Check sheet for the modelled part. Datum: model origin and axes. Units: mm. Round coordinates to 2 decimals unless told otherwise and drop trailing zeros.
Q1. Cross-section at A-A on y = 0.9. Give the number of separate pieces and of enclosed holes in the cut face, then the cut area to 3 significant figures.
Q2. Depth check by flat-ended pin: P1, Ø3.5, axis at x = -7.07, z = 7.07, coming from the +Y side; P2, Ø5.5, axis at x = -135, z = 0, coming from the -Y side. Enter the tip coordinate at first touch or a pass-through.
Q3. Scan lines: probe 1 along X at (y, z) = (0.4, -7.5); probe 2 along X at (y, z) = (0.35, 10); probe 3 along X at (y, z) = (1.3, -9). Record each from-to range of solid material in increasing order.
from build123d import *

# Parameters (mm, degrees)
SKETCH2_R           = 1.09
SKETCH2_R_2         = 3
SKETCH2_R_3         = 6.25
BOSS_EXTRUDE1_DEPTH = 1.5
FILLET1_R           = 10
SKETCH3_R           = 1.09
CUT_EXTRUDE1_DEPTH  = 10


with BuildPart() as part:
    # Sketch2 → Boss-Extrude1 (new body)
    with BuildSketch(Plane(origin=(0, 0, 0), x_dir=(1, 0, 0), z_dir=(0, 1, 0))):
        with BuildLine():
            add(Edge.make_bspline(
                [(15.330967743, -8.438686395), (-4.328656702, -48.917065398), (-54.77019988, -54.651995587)],
                knots=[0, 0, 0, 1, 1, 1], degree=2))
            ThreePointArc((15.330967743, -8.438686395), (3.221708095, 17.200889423), (-17.345753159, -2.318371704))
            add(Edge.make_bspline(
                [(-17.345753159, -2.318371704), (-24.57230847, -34.004755189), (-64.372079348, -27.287713928)],
                knots=[0, 0, 0, 1, 1, 1], degree=2))
            add(Edge.make_bspline(
                [(-118.261066558, 5.104714216), (-107.65521746, -9.024230402), (-84.042514499, -23.671917894), (-64.372079348, -27.287713928)],
                knots=[0, 0, 0, 0, 1, 1, 1, 1], degree=3))
            ThreePointArc((-118.261066558, 5.104714216), (-148.55197352, 11.072218102), (-136.664707239, -17.420641487))
            add(Edge.make_bspline(
                [(-136.664707239, -17.420641487), (-99.493020923, -49.665084924), (-54.77019988, -54.651995587)],
                knots=[0, 0, 0, 1, 1, 1], degree=2))
        make_face()
        with Locations(Location((-141.01040764, -6.01040764, 0), (0, 0, 270))):
            Circle(SKETCH2_R, mode=Mode.SUBTRACT)
        with Locations(Location((-128.98959236, -6.01040764, 0), (0, 0, 270))):
            Circle(SKETCH2_R, mode=Mode.SUBTRACT)
        with Locations(Location((-135, 0, 0), (0, 0, 270))):
            Circle(SKETCH2_R_2, mode=Mode.SUBTRACT)
        with Locations(Location((-141.01040764, 6.01040764, 0), (0, 0, 270))):
            Circle(SKETCH2_R, mode=Mode.SUBTRACT)
        with Locations(Location((-128.98959236, 6.01040764, 0), (0, 0, 270))):
            Circle(SKETCH2_R, mode=Mode.SUBTRACT)
        with Locations(Location((-7.071067812, -7.071067812, 0), (0, 0, 270))):
            Circle(SKETCH2_R, mode=Mode.SUBTRACT)
        with Locations(Location((7.071067812, -7.071067812, 0), (0, 0, 270))):
            Circle(SKETCH2_R, mode=Mode.SUBTRACT)
        with Locations(Location((-7.071067812, 7.071067812, 0), (0, 0, 270))):
            Circle(SKETCH2_R, mode=Mode.SUBTRACT)
        with Locations(Location((0, 0, 0), (0, 0, 270))):
            Circle(SKETCH2_R_3, mode=Mode.SUBTRACT)
        with Locations(Location((7.071067812, 7.071067812, 0), (0, 0, 270))):
            Circle(SKETCH2_R, mode=Mode.SUBTRACT)
    extrude(amount=BOSS_EXTRUDE1_DEPTH)

    # Fillet1
    fillet1_edges = [part.edges().sort_by_distance(p)[0] for p in [
        (-54.77019988, 0.75, 54.651995587),
    ]]
    fillet(fillet1_edges, radius=FILLET1_R)

    # Sketch3 → Cut-Extrude1 (cut)
    with BuildSketch(Plane(origin=(0, 1.5, 0), x_dir=(1, 0, 0), z_dir=(0, 1, 0))):
        with Locations(Location((-17.11634733, -28.475205037, 0), (0, 0, 270))):
            Circle(SKETCH3_R)
        with Locations(Location((-108.461839112, -21.891809685, 0), (0, 0, 270))):
            Circle(SKETCH3_R)
    extrude(amount=-CUT_EXTRUDE1_DEPTH, mode=Mode.SUBTRACT)


solid = part.part
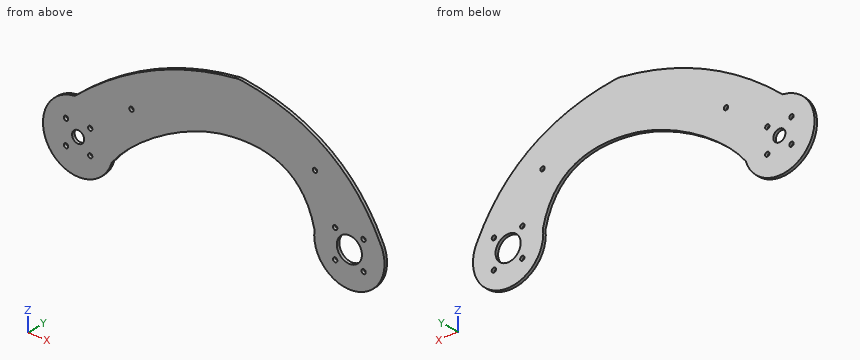
Results found:
1. separate pieces: 1
1. enclosed holes: 12
1. area: 5,270 mm2
2. P1: stops at y = 1.5
2. P2: passes through
3. probe 1: x = -150.81 to -119.19, -15.81 to -8.07, -6.07 to 6.07, 8.07 to 15.81
3. probe 2: x = -149.36 to -102.29, -19.81 to 14.55
3. probe 3: x = -150.01 to -119.99, -15.01 to 15.01
